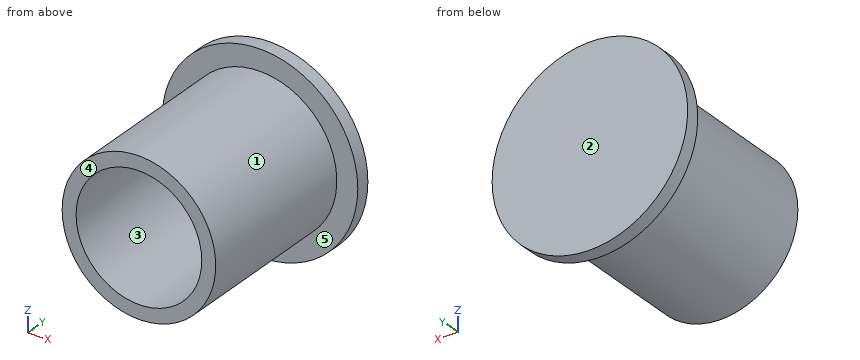
Autodesk Inventor part; units mm, degrees
ref_plane "YZ Plane" through (0, 0, 0) normal (1, 0, 0) x (0, 1, 0)
ref_plane "XZ Plane" through (0, 0, 0) normal (0, 1, 0) x (-1, 0, 0)
ref_plane "XY Plane" through (0, 0, 0) normal (0, 0, 1) x (1, 0, 0)
sketch "Szkic1" plane through (0, 0, 0) normal (0, 1, 0) x (-1, 0, 0)
  circle A0 centre (0, 0) radius 11
  circle A1 centre (0, 0) radius 9
  dimension "d0" = 22
  dimension "d1" = 2
extrude "Wyciągnięcie proste1" add sketch "Szkic1" along normal blind 24
sketch "Szkic2" plane through (0, 24, 0) normal (0, 1, 0) x (1, 0, 0)
  circle A0 centre (0, 0) radius 14
  circle A1 centre (0, 0) radius 11
  dimension "d4" = 28
  dimension "d7" = 3
extrude "Wyciągnięcie proste2" add sketch "Szkic2" along normal blind 2 contours A0 | A1
properties part number "tuleja"
Build history of the part. All positions in model axes, mm. Face numbers are marked on the shaded views. A direction names the side the tool comes from. Coordinates: 2 decimals unless noted, no trailing zeros. Write each loop counter-clockwise with the first axis right and the second up, starting at its lowest first coordinate (ties: lowest second). Pieces come first, ordered by that corner, then holes. Notation, with made-up numbers: (69, 31.25) -> (93, 31.25) arc R28 ccw to (93, 69.25) -> close; hole circle Ø7 at (-37.75, -19). An arc over 180 degrees is marked (long way). Use CSV: the item, a comma, the result in double quotes. Start each with the question number.
Q1. Pull direction X, two halves, no side cores. Call the marked faces 1, 2 and 3: released by +X, released by -X, zero draft, split by the parting line, or undercut.
Q2. Flat gauge pins, fed straight in: pin 1 Ø9 at (x, z) = (0, 2.5) entering from -Y; pin 2 Ø5 at (y, z) = (3, -3.5) entering from +X; pin 3 Ø3 at (y, z) = (18, -2.5) entering from -X. Where does each tip first touch, or does it go through?
Q3. 3-axis set-ups, long thin cutter, end or side, ignore diameter. For the marked faces 4 and 5: which of +Z, -Z, +X, -X, +Y, -Y reach the whole face in a straight line?
Q4. Cut at C-C, the plane y = 4.75. List the corners of the cut face in (x, z), then the cut area to 3 significant figures.
Q5. Cut at B-B, the plane x = 0. List the corners of the cut face in (y, z), then the cut area to 3 significant figures.
Q6. Cut at A-A, the plane z = 0. List the corners of the cut face in (x, y), then the cut area to 3 significant figures.
Q7. Cut at D-D, the plane x = 10.25. List the corners of the cut face in (y, z), then the cut area to 3 significant figures.
Q8. Drill centre lines: probe 1 along Z at (x, y) = (0, 19); probe 2 along Z at (x, y) = (-4.5, 17.5). Where is each one in solid material? Low to high.
Checked values:
1,face 1,"split by the parting line"
1,face 2,"zero draft"
1,face 3,"undercut"
2,pin 1,"stops at y = 24"
2,pin 2,"stops at x = 10.95"
2,pin 3,"stops at x = -10.95"
3,face 4,"+Z, -Z, +X, -X, -Y"
3,face 5,"-Y"
4,outline,"circle Ø22 at (0, 0); hole circle Ø18 at (0, 0)"
4,area,"126 mm²"
5,outline,"(0, -11) -> (24, -11) -> (24, -14) -> (26, -14) -> (26, 14) -> (24, 14) -> (24, 11) -> (0, 11) -> (0, 9) -> (24, 9) -> (24, -9) -> (0, -9) -> close"
5,area,"152 mm²"
6,outline,"(-14, 24) -> (-11, 24) -> (-11, 0) -> (-9, 0) -> (-9, 24) -> (9, 24) -> (9, 0) -> (11, 0) -> (11, 24) -> (14, 24) -> (14, 26) -> (-14, 26) -> close"
6,area,"152 mm²"
7,outline,"(0, -3.99) -> (24, -3.99) -> (24, -9.54) -> (26, -9.54) -> (26, 9.54) -> (24, 9.54) -> (24, 3.99) -> (0, 3.99) -> close"
7,area,"230 mm²"
8,probe 1,"z = -11 to -9, 9 to 11"
8,probe 2,"z = -10.04 to -7.79, 7.79 to 10.04"
